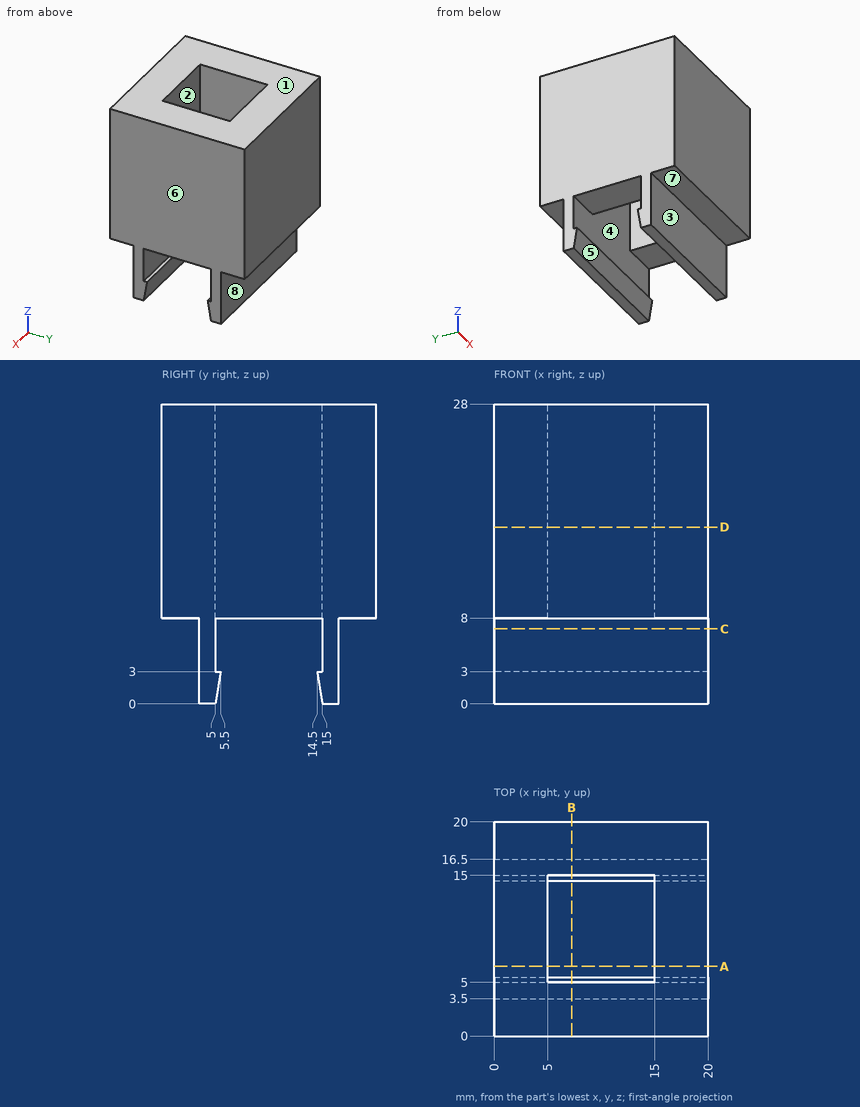
Print and shaded views of the part. All mm, measured from the part's lowest x, y and z. A direction names the side the tool comes from. Coordinates: 2 decimals unless noted, no trailing zeros. Loops run counter-clockwise (first coordinate to the right, second up) from the corner with the lowest first, then second, coordinate; pieces in that order, holes last. Notation, with made-up numbers: (-11, 25.25) -> (46, 25.25) arc R34 cw to (46, 59.25) -> close; hole circle Ø6 at (43.25, 10). An arc over 180 degrees is marked (long way). Use one line per item in the form item = value. Start each with the question number.
(1) Tool access for the marked faces 5, 6, 7 and 8: list every direction of +Z, -Z, +X, -X, +Y, -Y with a clear straight run to the whole face (end or side of a thin tool).
(2) Flat gauge pins, fed straight in: pin 1 (1.8 mm diameter, centred on x = 9.5, y = 2.5, fed in from -Z); pin 2 (5 mm diameter, centred on x = 4, z = 3, fed in from -Y); pin 3 (2.5 mm diameter, centred on x = 7.5, z = 6, fed in from +Y). Where does each tip first touch, or does it go through?
(3) Pull direction Z, two halves, no side cores. Call the marked faces 1, 2, 3 and 4: pulls with the +Z half, pulls with the -Z half, needs draft (parallel to the pull), parting line crosses it, or undercut.
(4) Cut at B-B on x = 7.25. Give the cut face in (y, z).
(5) Cut at D-D on z = 16.5. Give the cut face in (x, y), and give its area (3 significant figures).
(6) Cut at C-C on z = 7. Give the cut face in (x, y).
(7) Cut at A-A on y = 6.5. Give the cut face in (x, z).
(8) Probe probe 1 along Y at (x, z) = (18.75, 4); probe 2 along Y at (x, z) = (5.75, 20.25). List the from-to ranges inside material, lowest first. Write a range as from..to.
Values:
q1.face_5 = -Z, +X, -X
q1.face_6 = +Z, -Z, +X, +Y, -Y
q1.face_7 = -Z, +X, -X, -Y
q1.face_8 = -Z, +X, -X, +Y
q2.pin_1 = 8
q2.pin_2 = 3.5
q2.pin_3 = 16.5
q3.face_1 = pulls with the +Z half
q3.face_2 = undercut
q3.face_3 = needs draft
q3.face_4 = undercut
q4.outline = (0, 8) -> (3.5, 8) -> (3.5, 0) -> (5, 0) -> (5.5, 3) -> (5, 3) -> (5, 28) -> (0, 28) -> close; (14.5, 3) -> (15, 0) -> (16.5, 0) -> (16.5, 8) -> (20, 8) -> (20, 28) -> (15, 28) -> (15, 3) -> close
q5.outline = (0, 0) -> (20, 0) -> (20, 20) -> (0, 20) -> close; hole (5, 5) -> (15, 5) -> (15, 15) -> (5, 15) -> close
q5.area = 300 mm2
q6.outline = (0, 3.5) -> (20, 3.5) -> (20, 5) -> (0, 5) -> close; (0, 15) -> (20, 15) -> (20, 16.5) -> (0, 16.5) -> close
q7.outline = (0, 8) -> (5, 8) -> (5, 28) -> (0, 28) -> close; (15, 8) -> (20, 8) -> (20, 28) -> (15, 28) -> close
q8.probe_1 = 3.5..5, 15..16.5
q8.probe_2 = 0..5, 15..20
